Could you check a few things on this drawing? It's one solid part, dimensions in mm from its lowest x, y, z. A direction names the side the tool comes from. Give positions to 0.01 mm unless a question says otherwise; leave off trailing zeros. Write each loop counter-clockwise with the first axis right and the second up, starting at its lowest first coordinate (ties: lowest second). Pieces come first, ordered by that corner, then holes. Notation, with made-up numbers: M -10,87.5 L 10,87.5 A33 cw 10,116.5 Z; hole C 3.5,66.25 d1. An arc over 180 degrees is marked long. Use CSV: the item, a comma, the result in double quotes. Start each with the question number.
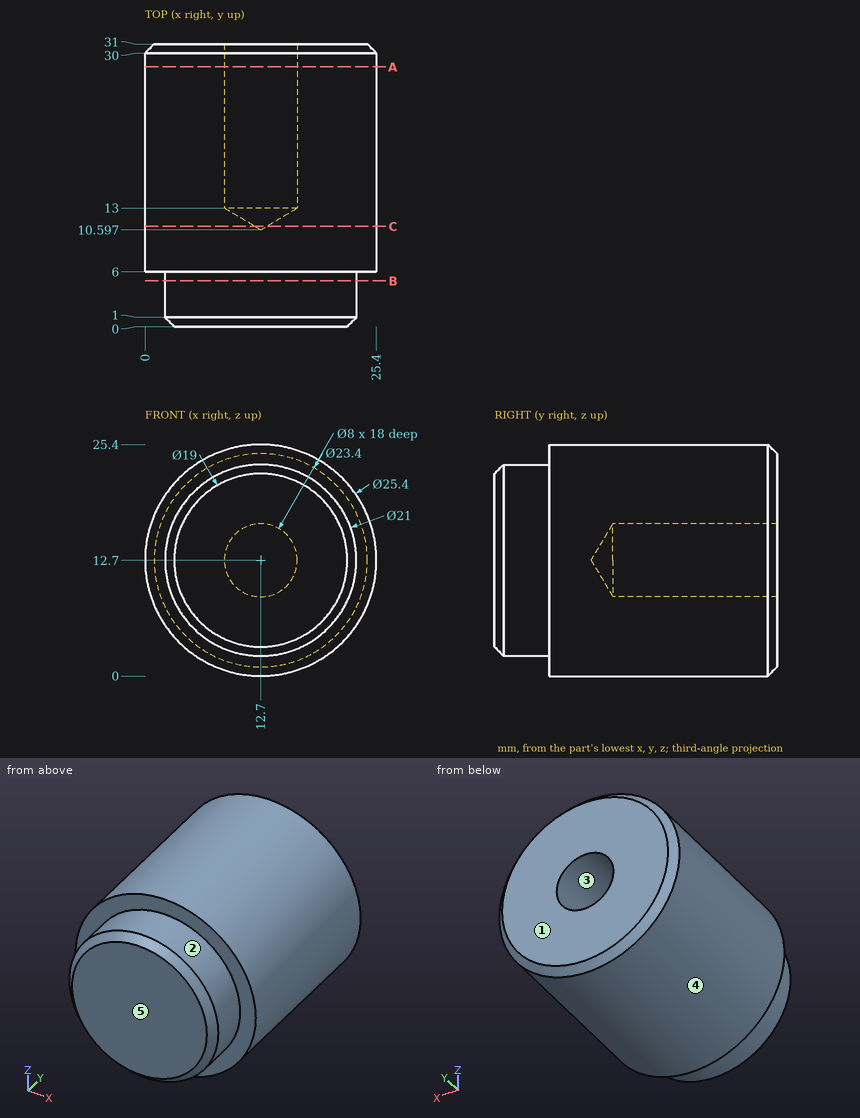
(1) I want a section at A-A (y = 28.5). Write out the boundary of the cut face in (x, z).
(2) I want a section at C-C (y = 11). Write out the boundary of the cut face in (x, z).
(3) Which directions (+Z, -Z, +X, -X, +Y, -Y) give clear straight access to the entire face, cutting with the end or side of a thin tool? Please do the marked faces 1 and 2.
(4) Will these pins go through, and if not, where does the flat tip stop? pin 1 Ø8 at (y, z) = (18, 17) entering from +X; pin 2 Ø1 at (x, z) = (15, 22.5) entering from -Y (1 decimal); pin 3 Ø3 at (x, y) = (15, 15.5) entering from +Z (1 decimal).
(5) I want a section at B-B (y = 5). Write out the boundary of the cut face in (x, z).
(6) Please list where these lines run through material, in increasing order: L1, parallel to Z at x = 12.7, y = 19; L2, parallel to Y at x = 6.5, z = 3.25. Write a range as [from, to].
(7) Thinking about a two-plate mould opening in Z: for the marked faces 3, 4 and 5, which applies, released by +Z, released by -Z, zero draft, split by the parting line, or undercut?
Geometry results:
1,outline,"C 12.7,12.7 d25.4; hole C 12.7,12.7 d8"
2,outline,"C 12.7,12.7 d25.4; hole C 12.7,12.7 d1.34"
3,face 1,"+Z, -Z, +X, -X, +Y"
3,face 2,"-Y"
4,pin 1,"stops at x = 25.4"
4,pin 2,"stops at y = 0.1"
4,pin 3,"stops at z = 25.4"
5,outline,"C 12.7,12.7 d21"
6,L1,"z = [0, 8.7], [16.7, 25.4]"
6,L2,"y = [6, 31]"
7,face 3,"undercut"
7,face 4,"split by the parting line"
7,face 5,"zero draft"
